Input: part model. Units: mm. Frame: model coordinates. Face numbers are marked on the shaded views. A direction names the side the tool comes from. Coordinates: 2 decimals unless noted, no trailing zeros. Order: outer loops, then holes, each group sorted by start corner. A loop starts at its lowest first (then second) coordinate and runs counter-clockwise, first axis right, second up.
from build123d import *

# Parameters (mm, degrees)
CIRPATTERN1_COUNT = 2
CIRPATTERN1_ANGLE = 90


with BuildPart() as part:
    # BodySke → Base-Revolve (revolve)
    with BuildSketch(Plane.XY, mode=Mode.PRIVATE) as base_revolve_sk:
        with BuildLine():
            Line((0, 0), (20.727669073, 0))
            Line((20.727669073, 0), (20.727669073, 1.5))
            Line((20.727669073, 1.5), (2.427669073, 1.5))
            Line((2.427669073, 1.5), (1.177669073, 2.75))
            Line((1.177669073, 2.75), (0.529956332, 2.75))
            ThreePointArc((0.529956332, 2.75), (0.133696843, 1.400299407), (0, 0))
        make_face()
    revolve(base_revolve_sk.sketch.rotate(Axis((-15.875, 0, 0), (1, 0, 0)), 90), axis=Axis((-15.875, 0, 0), (1, 0, 0)))

    # Sketch3 → Cross section 0
    with BuildSketch(Plane(origin=(0, 0, 0), x_dir=(0, 0, -1), z_dir=(1, 0, 0))):
        with BuildLine():
            Line((0.415, -1.72), (-0.415, -1.72))
            Line((-0.415, -1.72), (-0.415, 1.72))
            Line((-0.415, 1.72), (0.415, 1.72))
            Line((0.415, 1.72), (0.415, -1.72))
        make_face()
    # Sketch4 → Cross section 1
    with BuildSketch(Plane(origin=(2.33, 0, 0), x_dir=(0, 0, -1), z_dir=(1, 0, 0))):
        with BuildLine():
            Line((0.2075, -0.2075), (-0.2075, -0.2075))
            Line((-0.2075, -0.2075), (-0.2075, 0.2075))
            Line((-0.2075, 0.2075), (0.2075, 0.2075))
            Line((0.2075, 0.2075), (0.2075, -0.2075))
        make_face()
    cross = loft(mode=Mode.SUBTRACT)

    # CirPattern1: Cross ×2 about axis
    cirpattern1_axis = Axis((0, 0, 0), (1, 0, 0))
    for i in range(1, CIRPATTERN1_COUNT):
        add(cross.rotate(cirpattern1_axis, i * CIRPATTERN1_ANGLE / (CIRPATTERN1_COUNT - 1)), mode=Mode.SUBTRACT)


solid = part.part
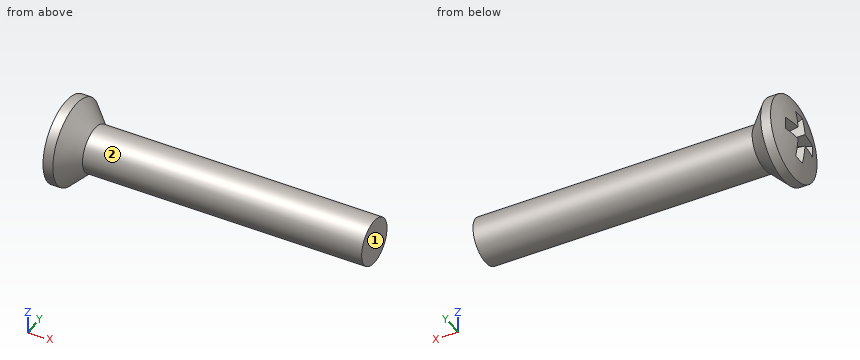
Item 1: Cut plane A-A on x = 8.5. Return loops of the section in (y, z), then the cut area to 3 significant figures.
Response values:
outline: circle Ø3 at (0, 0)
area: 7.07 mm2
Item 2: Pin query (flat end, axial travel): pin 1 Ø1.5 at (x, y) = (7.5, -0.5) entering from +Z; pin 2 Ø2 at (x, z) = (4.5, 2) entering from +Y. Return the tip coordinate at first contact, or that it passes through.
Response values:
pin 1: stops at z = 1.5
pin 2: stops at y = 1.12
Item 3: Access query for the marked faces 1 and 2. Directions: +Z, -Z, +X, -X, +Y, -Y. A direction counts if a zero-diameter tool reaches every point of the face in a straight line with its end or side. Return the directions, or none.
Response values:
face 1: +Z, -Z, +X, +Y, -Y
face 2: +X
Item 4: Ray query, probe 1 along Z at (x, y) = (12.5, -0.1); probe 2 along Z at (x, y) = (1.5, -0.2); probe 3 along X at (y, z) = (1.3, 2.05). Return the intervals inside material, ascending.
Response values:
probe 1: z = -1.5 to 1.5
probe 2: z = -2.42 to -0.75, 0.75 to 2.42
probe 3: x = 0.41 to 1.5
